```python
from build123d import *

# Parameters (mm, degrees)
SKETCH1_W           = 30
SKETCH1_H           = 5
BOSS_EXTRUDE1_DEPTH = 65
CUT_EXTRUDE1_DEPTH  = 81.015043264
SKETCH3_W           = 10
SKETCH3_H           = 5
BOSS_EXTRUDE2_DEPTH = 5
SKETCH4_W           = 1.25
SKETCH4_H           = 2.5
SKETCH4_W_2         = 3
SKETCH4_H_2         = 5
CUT_EXTRUDE2_DEPTH  = 85.127327002
SKETCH5_W           = 5
SKETCH5_H           = 15
CUT_EXTRUDE3_DEPTH  = 85.127327002


with BuildPart() as part:
    # Sketch1 → Boss-Extrude1 (new body)
    with BuildSketch(Plane.XY):
        with Locations((31.394042166, -137)):
            Rectangle(SKETCH1_W, SKETCH1_H)
    extrude(amount=BOSS_EXTRUDE1_DEPTH)

    # Sketch2 → Cut-Extrude1 (cut, through all)
    with BuildSketch(Plane.XZ.offset(139.5)):
        Polygon((21.144042166, 10), (24.144042166, 10), (24.144042166, 5), (25.394042166, 5), (25.394042166, 2.5), (24.144042166, 2.5), (24.144042166, 0), (21.144042166, 0), (21.144042166, 2.5), (19.894042166, 2.5), (19.894042166, 5), (21.144042166, 5), align=None)
        Polygon((41.644042166, 10), (38.644042166, 10), (38.644042166, 5), (37.394042166, 5), (37.394042166, 2.5), (38.644042166, 2.5), (38.644042166, 0), (41.644042166, 0), (41.644042166, 2.5), (42.894042166, 2.5), (42.894042166, 5), (41.644042166, 5), align=None)
    extrude(amount=-CUT_EXTRUDE1_DEPTH, mode=Mode.SUBTRACT)

    # Sketch3 → Boss-Extrude2 (add)
    with BuildSketch(Plane.XZ.offset(139.5)):
        with Locations((21.394042166, 67.5)):
            Rectangle(SKETCH3_W, SKETCH3_H)
        with Locations((41.394042166, 67.5)):
            Rectangle(SKETCH3_W, SKETCH3_H)
    extrude(amount=-BOSS_EXTRUDE2_DEPTH)

    # Sketch4 → Cut-Extrude2 (cut, through all)
    with BuildSketch(Plane.XZ.offset(139.5)):
        with Locations((29.269042166, 61.25)):
            Rectangle(SKETCH4_W, SKETCH4_H)
        with Locations((31.394042166, 63.75)):
            Rectangle(SKETCH4_W_2, SKETCH4_H)
        with Locations((31.394042166, 61.25)):
            Rectangle(SKETCH4_W_2, SKETCH4_H)
        with Locations((31.394042166, 57.5)):
            Rectangle(SKETCH4_W_2, SKETCH4_H_2)
        with Locations((33.519042166, 61.25)):
            Rectangle(SKETCH4_W, SKETCH4_H)
    extrude(amount=-CUT_EXTRUDE2_DEPTH, mode=Mode.SUBTRACT)

    # Sketch5 → Cut-Extrude3 (cut, through all)
    with BuildSketch(Plane(origin=(0, -134.5, 0), x_dir=(1, 0, 0), z_dir=(0, 1, 0))):
        with Locations((41.394042166, -62.5)):
            Rectangle(SKETCH5_W, SKETCH5_H)
    extrude(amount=-CUT_EXTRUDE3_DEPTH, mode=Mode.SUBTRACT)


solid = part.part
```
Check sheet for the modelled part. Datum: model origin and axes. Units: mm. A direction names the side the tool comes from. Coordinates: 2 decimals unless noted, no trailing zeros. Write each loop counter-clockwise with the first axis right and the second up, starting at its lowest first coordinate (ties: lowest second). Pieces come first, ordered by that corner, then holes. Notation, with made-up numbers: M 28,3 L 69,3 A22 ccw 69,19 Z; hole C 44.25,-29 d2. An arc over 180 degrees is marked long. Use one line per item in the form item = value.
Item 1: Set-up check for faces 4 (the face through (38.644, -137, 8)), 5 (the face through (46.394, -137, 35)), 6 (the face through (42.894, -137, 4)), 7 (the face through (44, -137, 0)), 8 (the face through (32.894, -137, 64)): record each of +Z, -Z, +X, -X, +Y, -Y from which the full face is reachable in a straight line by a thin tool's end or side.
Answer below:
face_4 = -Z, +Y, -Y
face_5 = +Z, -Z, +X, +Y, -Y
face_6 = +Y, -Y
face_7 = -Z, +X, -X, +Y, -Y
face_8 = +Z, +Y, -Y
Item 2: Release check for a two-part mould opening along Z. For faces 1 (the face through (21.144, -137, 1)), 2 (the face through (21, -137, 70)), 3 (the face through (37.394, -137, 4)) record: pulls with the +Z half, pulls with the -Z half, needs draft (parallel to the pull), parting line crosses it, or undercut.
Answer below:
face_1 = needs draft
face_2 = pulls with the +Z half
face_3 = undercut
Item 3: Sectioned sample at A-A, the plane z = 6. Record the cut outline in (x, y), and give its area (3 significant figures).
Answer below:
outline = M 16.39,-139.5 L 21.14,-139.5 L 21.14,-134.5 L 16.39,-134.5 Z; M 24.14,-139.5 L 38.64,-139.5 L 38.64,-134.5 L 24.14,-134.5 Z; M 41.64,-139.5 L 46.39,-139.5 L 46.39,-134.5 L 41.64,-134.5 Z
area = 120 mm^2
Item 4: Sectioned sample at C-C, the plane x = 23.5. Record the cut outline in (y, z), and give its area (3 significant figures).
Answer below:
outline = M -139.5,10 L -134.5,10 L -134.5,70 L -139.5,70 Z
area = 300 mm^2
Item 5: Sectioned sample at B-B, the plane z = 58. Record the cut outline in (x, y).
Answer below:
outline = M 16.39,-139.5 L 29.89,-139.5 L 29.89,-134.5 L 16.39,-134.5 Z; M 32.89,-139.5 L 38.89,-139.5 L 38.89,-134.5 L 32.89,-134.5 Z; M 43.89,-139.5 L 46.39,-139.5 L 46.39,-134.5 L 43.89,-134.5 Z
Item 6: Sectioned sample at D-D, the plane x = 27.5. Record the cut outline in (y, z).
Answer below:
outline = M -139.5,0 L -134.5,0 L -134.5,65 L -139.5,65 Z
Item 7: Gauge pin test, flat ends, axial feed: pin 1 Ø1 at (x, y) = (39.5, -138.5) entering from +Z; pin 2 Ø1 at (x, y) = (33, -138) entering from +Z; pin 3 Ø1.5 at (x, y) = (27, -138.5) entering from +Z; pin 4 Ø2.5 at (x, y) = (22.5, -136) entering from -Z. Record the tip position at first contact, or that the pin passes through.
Answer below:
pin_1 = 55
pin_2 = 65
pin_3 = 70
pin_4 = 10
Item 8: Material ranges on L1, parallel to X at y = -137.55, z = 55.5; L2, parallel to Z at x = 37.5, y = -138.15; L3, parallel to Z at x = 28.75, y = -136.8, recorded low to high. Write a range as from..to.
Answer below:
L1 = 16.39..29.89, 32.89..38.89, 43.89..46.39
L2 = 0..2.5, 5..70
L3 = 0..60, 62.5..65
